Autodesk Inventor part; units mm, degrees
ref_plane "YZ Plane" through (0, 0, 0) normal (1, 0, 0) x (0, 1, 0)
ref_plane "XZ Plane" through (0, 0, 0) normal (0, 1, 0) x (-1, 0, 0)
ref_plane "XY Plane" through (0, 0, 0) normal (0, 0, 1) x (1, 0, 0)
sketch "スケッチ1" plane through (0, 0, 0) normal (0, 1, 0) x (-1, 0, 0)
  circle A0 centre (0, 0) radius 12.5
  dimension "d0" = 25
extrude "押し出し1" add sketch "スケッチ1" along normal blind 2
sketch "スケッチ2" plane through (0, 2, 0) normal (0, 1, 0) x (1, 0, 0)
  circle A0 centre (0, 0) radius 12.5
  circle A1 centre (0, 0) radius 10
  dimension "d3" = 25
  dimension "d4" = 20
extrude "押し出し2" add sketch "スケッチ2" along normal blind 17
sketch "スケッチ3" plane through (0, 2, 0) normal (0, 1, 0) x (1, 0, 0)
  arc A0 (-6.4279, -7.6604) -> (0, -10) centre (0, 0) ccw
  line L0 (0, 0) -> (-6.4279, -7.6604) construction
  line L1 (0, 0) -> (0, -10) construction
  arc A1 (6.4279, 7.6604) -> (0, 10) centre (0, 0) ccw
  line L2 (0, 0) -> (6.4279, 7.6604) construction
  line L3 (0, 0) -> (0, 10) construction
  circle A2 centre (0, 0) radius 10
  line L4 (-6.4279, -7.6604) -> (0, 0)
  line L5 (0, 0) -> (6.4279, 7.6604)
  line L6 (0, -10) -> (0, 0)
  line L7 (0, 10) -> (0, 0)
  circle A3 centre (0, 0) radius 10
  point P0 (3.2139, 3.8302)
  dimension "d8" = 40
  dimension "d10" = 40
  dimension "d11" = 3.8302
  dimension "d12" = 6.4279
extrude "押し出し3" add sketch "スケッチ3" along normal blind 6.5 contours L4 L6 A0 | A1 L5 L7
sketch "スケッチ4" plane through (0, 8.5, 0) normal (0, 1, 0) x (1, 0, 0)
  line L0 (0, -10) -> (0, 0)
  circle A0 centre (0, 0) radius 1
  dimension "d15" = 2
extrude "押し出し4" cut sketch "スケッチ4" against normal blind 7
ref_plane "作業平面1" through (0, 9, 0) normal (0, 1, 0) x (1, 0, 0)
sketch "スケッチ5" plane through (0, 8.5, 0) normal (0, 1, 0) x (1, 0, 0)
  line L0 (0, -10) -> (0, -1)
  arc A0 (0, -10) -> (6.4279, -7.6604) centre (0, 0) ccw
  line L1 (0, 0) -> (6.4279, -7.6604) construction
  line L2 (0, 0) -> (0, -10) construction
  arc A1 (0, -8) -> (4, -6.9282) centre (0, 0) ccw
  line L3 (0, 0) -> (4, -6.9282) construction
  line L4 (0, 0) -> (0, -8) construction
  arc A2 (3.5, -6.0622) -> (4.4995, -5.3623) centre (0, 0) ccw
  line L5 (0, 0) -> (4.4995, -5.3623) construction
  line L6 (0, 0) -> (3.5, -6.0622) construction
  arc A3 (0, -10) -> (6.4279, 7.6604) centre (0, 0) ccw
  line L7 (0, -10) -> (0, -8)
  line L8 (6.4279, -7.6604) -> (4.4995, -5.3623)
  line L9 (4, -6.9282) -> (3.5, -6.0622)
  line L10 (0, 1) -> (0, 10)
  arc A4 (0, 10) -> (-6.4279, 7.6604) centre (0, 0) ccw
  line L11 (0, 0) -> (-6.4279, 7.6604) construction
  line L12 (0, 0) -> (0, 10) construction
  arc A5 (0, 8) -> (-4, 6.9282) centre (0, 0) ccw
  line L13 (0, 0) -> (-4, 6.9282) construction
  line L14 (0, 0) -> (0, 8) construction
  arc A6 (-3.5, 6.0622) -> (-4.4995, 5.3623) centre (0, 0) ccw
  line L15 (0, 0) -> (-3.5, 6.0622) construction
  line L16 (0, 0) -> (-4.4995, 5.3623) construction
  line L17 (-6.4279, 7.6604) -> (-4.4995, 5.3623)
  line L18 (-4, 6.9282) -> (-3.5, 6.0622)
  line L19 (0, 10) -> (0, 8)
  dimension "d19" = 10
  dimension "d20" = 40
  dimension "d21" = 8
  dimension "d22" = 30
  dimension "d23" = 7
  dimension "d24" = 10
  dimension "d25" = 10
  dimension "d26" = 40
  dimension "d27" = 8
  dimension "d28" = 30
  dimension "d29" = 7
  dimension "d30" = 10
extrude "押し出し5" add sketch "スケッチ5" against normal blind 5
fillet "フィレット1" radius 1 1 edges at (-4.4995, 6, -5.3623)
fillet "フィレット2" radius 1 1 edges at (4.4995, 6, 5.3623)
properties part number "kumi2"
Verification items for the finished model (mm, model axes). A direction names the side the tool comes from. Round coordinates to 2 decimals unless told otherwise and drop trailing zeros. Order: outer loops, then holes, each group sorted by start corner. A loop starts at its lowest first (then second) coordinate and runs counter-clockwise, first axis right, second up.
1) Cross-section at C-C, the plane y = 15. Record the cut outline in (x, z).
Geometry says:
outline: circle Ø25 at (0, 0); hole circle Ø20 at (0, 0)
2) Depth check by flat-ended pin: pin 1 (3 mm diameter, centred on x = 0.5, z = -4, fed in from +Y); pin 2 (3 mm diameter, centred on x = 7, z = 1.5, fed in from +Y); pin 3 (1 mm diameter, centred on x = 9, y = 13, fed in from -Z). Enter the tip coordinate at first touch or a pass-through.
Geometry says:
pin 1: stops at y = 8.5
pin 2: stops at y = 2
pin 3: stops at z = -9.17
3) Cross-section at B-B, the plane z = -3. Record the cut outline in (x, y), plus the area to 3 significant figures.
Geometry says:
outline: (-12.13, 0) - (12.13, 0) - (12.13, 19) - (9.54, 19) - (9.54, 2) - (2.52, 2) - (2.52, 8.5) - (0, 8.5) - (0, 2) - (-9.54, 2) - (-9.54, 19) - (-12.13, 19) - close
area: 153 mm2
4) Draft check along X on faces 4 (the flat face through (-5.774, 6.035, -6.881)), 5 (the cylindrical face through (0.824, 9.367, 12.473)), 6 (the flat face through (-0.1, 19, -10.2)). Enter one of: +X half, -X half, draft (parallel to the pull), parting line (faces both ways), or undercut.
Geometry says:
face 4: undercut
face 5: parting line
face 6: draft
5) Cross-section at A-A, the plane y = 4.5. Record the cut outline in (x, z).
Geometry says:
outline: circle Ø25 at (0, 0); hole (-6.43, -7.66) - (-5.1, -6.08) arc R1 cw to (-3.79, -5.88) arc R7 ccw to (-3.5, -6.06) - (-4, -6.93) arc R8 ccw to (0, -8) - (0, -1) arc R1 ccw to (0.64, -0.77) - (6.43, -7.66) arc R10 ccw to (6.43, 7.66) - (5.1, 6.08) arc R1 cw to (3.79, 5.88) arc R7 ccw to (3.5, 6.06) - (4, 6.93) arc R8 ccw to (0, 8) - (0, 1) arc R1 ccw to (-0.64, 0.77) - (-6.43, 7.66) arc R10 ccw to start
6) Material ranges on line 1 (Z direction, x = 0, y = 11.75); line 2 (X direction, y = 2.75, z = -2.5), recorded low to high.
Geometry says:
line 1: z = -12.5 to -10, 10 to 12.5
line 2: x = -12.25 to -9.68, 0 to 2.1, 9.68 to 12.25
7) Tool access check on faces 1 (the flat face through (3, 3.5, 8)), 2 (the flat face through (0, 0, 0)), 3 (the flat face through (3.49, 5.2, -4.16)). Record the directions out of +Z, -Z, +X, -X, +Y, -Y that give a thin tool (end or side, any length) a straight path to the whole face; none if there is none.
Geometry says:
face 1: none
face 2: +Z, -Z, +X, -X, -Y
face 3: +Y
